```python
from build123d import *

# Parameters (mm, degrees)
SKETCH_2_R          = 17.5
SKETCH_2_R_2        = 15
SKETCH_2_W          = 10
SKETCH_2_H          = 5
EXTRUDE_1_DEPTH     = 10
EXTRUDE_START       = 10
EXTRUDE_2_DEPTH     = 10
SKETCH_4_R          = 15
EXTRUDE_3_DEPTH     = 10
SKETCH_5_R          = 4.55
CUT_EXTRUDE_1_DEPTH = 43.804789452
SKETCH_6_R          = 1.5
CUT_EXTRUDE_2_DEPTH = 56.213223054
SKETCH_7_R          = 15
CUT_EXTRUDE_3_DEPTH = 13
CUT_EXTRUDE_START   = -3
SKETCH_8_R          = 15
CUT_EXTRUDE_4_DEPTH = 3
SKETCH_10_W         = 10
SKETCH_10_H         = 30
SKETCH_10_R         = 1.5
EXTRUDE_5_DEPTH     = 45
EXTRUDE_6_REACH     = 62.467
SKETCH_11_W         = 35
SKETCH_11_H         = 30
SKETCH_12_R         = 15
EXTRUDE_7_DEPTH     = 3
EXTRUDE_START_2     = -3
SKETCH_14_R         = 15
EXTRUDE_9_DEPTH     = 3
SKETCH_16_R         = 4.55
CUT_EXTRUDE_6_DEPTH = 20
SKETCH_15_W         = 55
SKETCH_15_H         = 30
CUT_EXTRUDE_7_DEPTH = 25


with BuildPart() as part:
    # Sketch 2 → Extrude 1 (new body)
    # profile 1 of 4: a face of its own
    with BuildSketch(Plane.XY):
        with BuildLine():
            ThreePointArc((-17.5, 0), (0, 17.5), (17.5, 0))
            Line((17.5, 0), (17.5, 17.5))
            Line((17.5, 17.5), (17.5, 21))
            Line((17.5, 21), (17.5, 26))
            Line((17.5, 26), (-17.5, 26))
            Line((-17.5, 26), (-17.5, 21))
            Line((-17.5, 21), (-17.5, 0))
        make_face()
    # profile 2 of 4: a face of its own
    with BuildSketch(Plane.XY):
        Circle(SKETCH_2_R)
        Circle(SKETCH_2_R_2, mode=Mode.SUBTRACT)
    # profile 3 of 4: a face of its own
    with BuildSketch(Plane.XY):
        with Locations((22.5, 23.5)):
            Rectangle(SKETCH_2_W, SKETCH_2_H)
    # profile 4 of 4: a face of its own
    with BuildSketch(Plane.XY):
        with Locations((-22.5, 23.5)):
            Rectangle(SKETCH_2_W, SKETCH_2_H)
    extrude(amount=EXTRUDE_1_DEPTH)

    # Sketch 3 → Extrude 2 (add)
    with BuildSketch(Plane(origin=(0, 0, 0), x_dir=(-1, 0, 0), z_dir=(0, 0, -1)).offset(EXTRUDE_START)):
        with BuildLine():
            Line((17.5, 0), (17.5, 21))
            Line((17.5, 21), (27.5, 21))
            Line((27.5, 21), (27.5, 26))
            Line((27.5, 26), (-27.5, 26))
            Line((-27.5, 26), (-27.5, 21))
            Line((-27.5, 21), (-17.5, 21))
            Line((-17.5, 21), (-17.5, 0))
            ThreePointArc((-17.5, 0), (0, -17.5), (17.5, 0))
        make_face()
    extrude(amount=-EXTRUDE_2_DEPTH)

    # Sketch 4 → Extrude 3 (add)
    with BuildSketch(Plane(origin=(0, 0, -10), x_dir=(-1, 0, 0), z_dir=(0, 0, -1)).offset(EXTRUDE_START)):
        with BuildLine():
            Line((17.5, 0), (17.5, 21))
            Line((17.5, 21), (27.5, 21))
            Line((27.5, 21), (27.5, 26))
            Line((27.5, 26), (-27.5, 26))
            Line((-27.5, 26), (-27.5, 21))
            Line((-27.5, 21), (-17.5, 21))
            Line((-17.5, 21), (-17.5, 0))
            ThreePointArc((-17.5, 0), (0, -17.5), (17.5, 0))
        make_face()
        with Locations(Location((0, 0, 0), (0, 0, 180))):
            Circle(SKETCH_4_R, mode=Mode.SUBTRACT)
    extrude(amount=-EXTRUDE_3_DEPTH)

    # Sketch 5 → Cut-Extrude 1 (cut, through all)
    with BuildSketch(Plane.XY):
        Circle(SKETCH_5_R)
    extrude(amount=-CUT_EXTRUDE_1_DEPTH, mode=Mode.SUBTRACT)

    # Sketch 6 → Cut-Extrude 2 (cut, through all)
    with BuildSketch(Plane(origin=(0, 26, 0), x_dir=(1, 0, 0), z_dir=(0, 1, 0))):
        with Locations(Location((-22.5, 15, 0), (0, 0, 270))):
            Circle(SKETCH_6_R)
        with Locations(Location((-22.5, -5, 0), (0, 0, 270))):
            Circle(SKETCH_6_R)
        with Locations(Location((22.5, 15, 0), (0, 0, 270))):
            Circle(SKETCH_6_R)
        with Locations(Location((22.5, -5, 0), (0, 0, 270))):
            Circle(SKETCH_6_R)
    extrude(amount=-CUT_EXTRUDE_2_DEPTH, mode=Mode.SUBTRACT)

    # Sketch 7 → Cut-Extrude 3 (cut)
    with BuildSketch(Plane(origin=(0, 0, -20), x_dir=(-1, 0, 0), z_dir=(0, 0, -1))):
        with Locations(Location((0, 0, 0), (0, 0, 180))):
            Circle(SKETCH_7_R)
    extrude(amount=-CUT_EXTRUDE_3_DEPTH, mode=Mode.SUBTRACT)

    # Sketch 8 → Cut-Extrude 4 (cut)
    with BuildSketch(Plane.XY.offset(CUT_EXTRUDE_START)):
        Circle(SKETCH_8_R)
    extrude(amount=CUT_EXTRUDE_4_DEPTH, mode=Mode.SUBTRACT)

    # Sketch 10 → Extrude 5 (add)
    # profile 1 of 2: a face of its own
    with BuildSketch(Plane.XZ.offset(-21)):
        with Locations((22.5, -5)):
            Rectangle(SKETCH_10_W, SKETCH_10_H)
        with Locations(Location((22.5, -15, 0), (0, 0, 90))):
            Circle(SKETCH_10_R, mode=Mode.SUBTRACT)
        with Locations(Location((22.5, 5, 0), (0, 0, 90))):
            Circle(SKETCH_10_R, mode=Mode.SUBTRACT)
    # profile 2 of 2: a face of its own
    with BuildSketch(Plane.XZ.offset(-21)):
        with Locations((-22.5, -5)):
            Rectangle(SKETCH_10_W, SKETCH_10_H)
        with Locations(Location((-22.5, 5, 0), (0, 0, 90))):
            Circle(SKETCH_10_R, mode=Mode.SUBTRACT)
        with Locations(Location((-22.5, -15, 0), (0, 0, 90))):
            Circle(SKETCH_10_R, mode=Mode.SUBTRACT)
    extrude(amount=EXTRUDE_5_DEPTH)

    # Sketch 11 → Extrude 6 (add, up to next)
    with BuildSketch(Plane.XZ.offset(24), mode=Mode.PRIVATE) as extrude_6_sk1:
        with Locations((0, -5)):
            Rectangle(SKETCH_11_W, SKETCH_11_H)
    extrude_6_tool1 = extrude(extrude_6_sk1.sketch, amount=-EXTRUDE_6_REACH, mode=Mode.PRIVATE) - part.part
    add(extrude_6_tool1.solids().sort_by_distance((0, -24, -5))[0])

    # Sketch 12 → Extrude 7 (add)
    with BuildSketch(Plane(origin=(0, 0, -20), x_dir=(-1, 0, 0), z_dir=(0, 0, -1))):
        Circle(SKETCH_12_R)
    extrude(amount=-EXTRUDE_7_DEPTH)

    # Sketch 14 → Extrude 9 (add)
    with BuildSketch(Plane.XY.offset(10).offset(EXTRUDE_START_2)):
        Circle(SKETCH_14_R)
    extrude(amount=EXTRUDE_9_DEPTH)

    # Sketch 16 → Cut-Extrude 6 (cut)
    with BuildSketch(Plane.XY.offset(10)):
        Circle(SKETCH_16_R)
    extrude(amount=-CUT_EXTRUDE_6_DEPTH, mode=Mode.SUBTRACT)

    # Sketch 15 → Cut-Extrude 7 (cut)
    with BuildSketch(Plane.XZ.offset(24)):
        with Locations((0, -5)):
            Rectangle(SKETCH_15_W, SKETCH_15_H)
    extrude(amount=-CUT_EXTRUDE_7_DEPTH, mode=Mode.SUBTRACT)


solid = part.part
```
Check sheet for the modelled part. Datum: model origin and axes. Units: mm. A direction names the side the tool comes from. Round coordinates to 2 decimals unless told otherwise and drop trailing zeros. Loops run counter-clockwise (first coordinate to the right, second up) from the corner with the lowest first, then second, coordinate; pieces in that order, holes last. Notation, with made-up numbers: (-13, 42.25) -> (26, 42.25) arc R36 cw to (26, 77.25) -> close; hole circle Ø9 at (61, -26.5). An arc over 180 degrees is marked (long way). Answer in a Markdown table with one row per item.
Q1. Sectioned sample at D-D on y = 9.75. Enter the section's corners in (x, z), then the cut area to 3 significant figures.
Data:
| item | result |
|---|---|
| outline | (-27.5, -20) -> (27.5, -20) -> (27.5, 10) -> (-27.5, 10) -> close; hole circle Ø3 at (-22.5, -15); hole circle Ø3 at (-22.5, 5); hole (-11.4, -17) -> (11.4, -17) -> (11.4, -7) -> (-11.4, -7) -> close; hole (-11.4, -3) -> (11.4, -3) -> (11.4, 7) -> (-11.4, 7) -> close; hole circle Ø3 at (22.5, -15); hole circle Ø3 at (22.5, 5) |
| area | 1,170 mm^2 |
Q2. Sectioned sample at A-A on x = 22.5. Enter the section's corners in (y, z).
Data:
| item | result |
|---|---|
| outline | (1, -20) -> (26, -20) -> (26, -16.5) -> (1, -16.5) -> close; (1, -13.5) -> (26, -13.5) -> (26, 3.5) -> (1, 3.5) -> close; (1, 6.5) -> (26, 6.5) -> (26, 10) -> (1, 10) -> close |
Q3. Release check for a two-part mould opening along Z. For faces 4 (the face through (0, 14, -20)), 5 (the face through (0, 15, -12)), 6 (the face through (21.49, 13.68, -16.11)), 7 (the face through (0.09, 4.55, 8.52)) record: released by +Z, released by -Z, zero draft, split by the parting line, or undercut.
Data:
| item | result |
|---|---|
| face 4 | released by -Z |
| face 5 | undercut |
| face 6 | undercut |
| face 7 | zero draft |
Q4. Set-up check for faces 1 (the face through (0, 15, 2)), 2 (the face through (-27.5, 14, -5)), 3 (the face through (0.09, 4.55, -4.97)): record each of +Z, -Z, +X, -X, +Y, -Y from which the full face is reachable in a straight line by a thin tool's end or side.
Data:
| item | result |
|---|---|
| face 1 | -Y |
| face 2 | +Z, -Z, -X, +Y, -Y |
| face 3 | +Z, -Y |
Q5. Thickness scan on L1, parallel to X at y = 17.25, z = -15; L2, parallel to Z at x = 3, y = 11.75; L3, parallel to Z at x = -22, y = 13.5. Record the ranges inside material, lowest first.
Data:
| item | result |
|---|---|
| L1 | x = -27.5 to -24, -21 to 21, 24 to 27.5 |
| L2 | z = -20 to -17, -7 to -3, 7 to 10 |
| L3 | z = -20 to -16.41, -13.59 to 3.59, 6.41 to 10 |
Q6. Sectioned sample at B-B on z = 5. Enter the section's corners in (x, y).
Data:
| item | result |
|---|---|
| outline | (-27.5, 1) -> (-24, 1) -> (-24, 26) -> (-27.5, 26) -> close; (-21, 1) -> (-14.97, 1) arc R15 cw to (14.97, 1) -> (21, 1) -> (21, 26) -> (-21, 26) -> close; (24, 1) -> (27.5, 1) -> (27.5, 26) -> (24, 26) -> close |
Q7. Sectioned sample at C-C on y = 24. Enter the section's corners in (x, z).
Data:
| item | result |
|---|---|
| outline | (-27.5, -20) -> (27.5, -20) -> (27.5, 10) -> (-27.5, 10) -> close; hole circle Ø3 at (-22.5, -15); hole circle Ø3 at (-22.5, 5); hole circle Ø3 at (22.5, -15); hole circle Ø3 at (22.5, 5) |
Q8. Go/stop test with flat-tipped pins: P1, Ø4, axis at x = -22.5, z = -15, coming from the +Y side; P2, Ø1, axis at x = 13, z = -9.5, coming from the -Y side; P3, Ø2.5, axis at x = 22.5, z = -15, coming from the -Y side (3 decimals). Record where each tip stops, or that it passes through.
Data:
| item | result |
|---|---|
| P1 | stops at y = 26 |
| P2 | stops at y = 6.54 |
| P3 | passes through |
